Geometry check sheet. Reference: drawing and pictorial views, mm from the part's lowest x, y, z. A direction names the side the tool comes from. Give positions to 0.01 mm unless a question says otherwise; leave off trailing zeros. Loops run counter-clockwise (first coordinate to the right, second up) from the corner with the lowest first, then second, coordinate; pieces in that order, holes last. Notation, with made-up numbers: M 20,-12 L 72,-12 A23 cw 72,24 Z; hole C 64,77.5 d5. An arc over 180 degrees is marked long. Put each result on its own line as item: value. Start each with the question number.
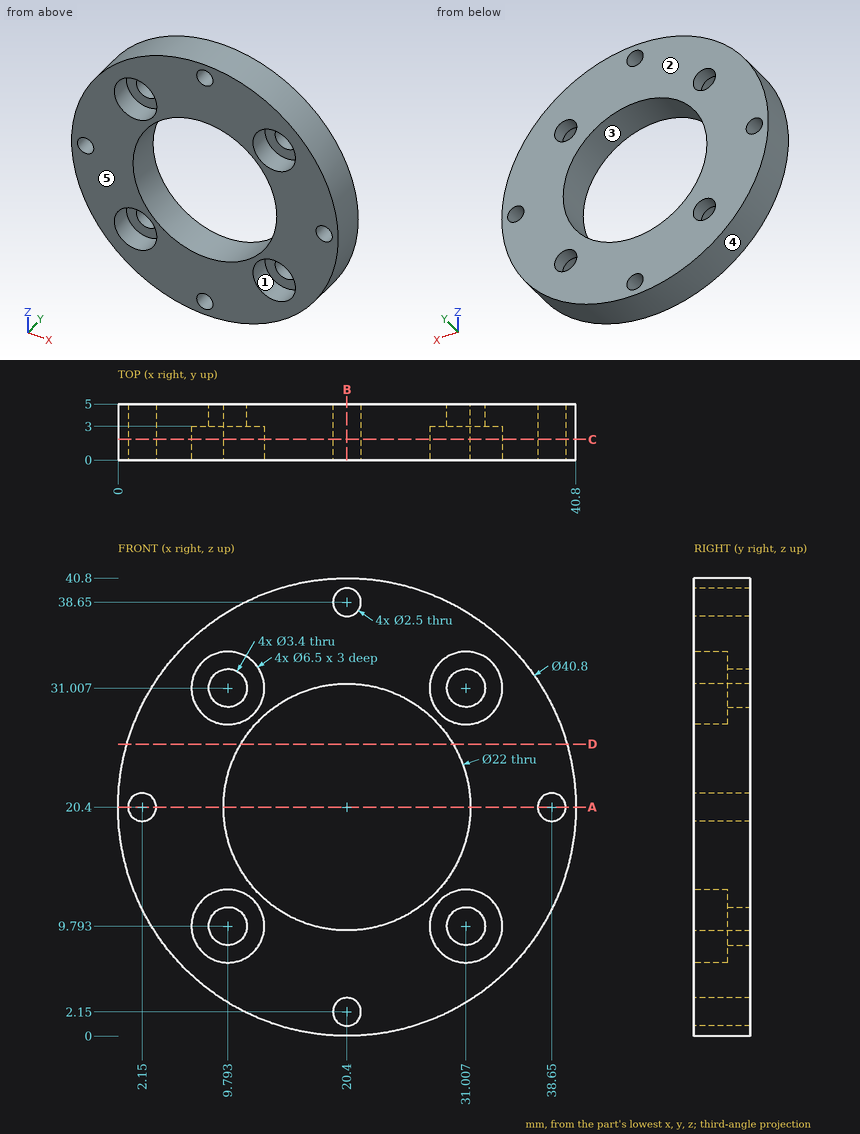
Q1. Section check B-B, the plane x = 20.4. Record the cut outline in (y, z).
Q2. Section check A-A, the plane z = 20.4. Record the cut outline in (x, y).
Q3. Mould release check, pull along Z, two halves, no side actions. Record for the marked faces 3, 4 and 5: pulls with the +Z half, pulls with the -Z half, needs draft (parallel to the pull), parting line crosses it, or undercut.
Q4. Depth check by flat-ended pin: P1, Ø4.5, axis at x = 31.01, z = 9.79, coming from the -Y side; P2, Ø3, axis at y = 4, z = 9.5, coming from the +X side (1 decimal); P3, Ø3, axis at y = 3, z = 14, coming from the -X side. Enter the tip coordinate at first touch or a pass-through.
Q5. Section check D-D, the plane z = 26. Record the cut outline in (x, y).
Q6. Thickness scan on line 1 along X through (y, z) = (3.15, 20.4); line 2 along Z through (x, y) = (7, 2.9) (1 decimal). Record the ranges inside material, lowest first. Write a range as [from, to].
Q7. Access from +Z, -Z, +X, -X, +Y, -Y to the whole of each face (thin tool, end or side, straight path). Record for the marked faces 1 and 2.
Q8. Section check C-C, the plane y = 1.85. Give the number of separate pieces and of enclosed holes in the cut face, then the cut area to 3 significant figures.
Found:
1. outline: M 0,0 L 5,0 L 5,0.9 L 0,0.9 Z; M 0,3.4 L 5,3.4 L 5,9.4 L 0,9.4 Z; M 0,31.4 L 5,31.4 L 5,37.4 L 0,37.4 Z; M 0,39.9 L 5,39.9 L 5,40.8 L 0,40.8 Z
2. outline: M 0,0 L 0.9,0 L 0.9,5 L 0,5 Z; M 3.4,0 L 9.4,0 L 9.4,5 L 3.4,5 Z; M 31.4,0 L 37.4,0 L 37.4,5 L 31.4,5 Z; M 39.9,0 L 40.8,0 L 40.8,5 L 39.9,5 Z
3. face 3: undercut
3. face 4: parting line crosses it
3. face 5: needs draft
4. P1: stops at y = 3
4. P2: stops at x = 38.5
4. P3: stops at x = 0.6
5. outline: M 0.78,0 L 10.93,0 L 10.93,5 L 0.78,5 Z; M 29.87,0 L 40.02,0 L 40.02,5 L 29.87,5 Z
6. line 1: x = [0, 0.9], [3.4, 9.4], [31.4, 37.4], [39.9, 40.8]
6. line 2: z = [5, 8.1], [11.5, 29.3], [32.7, 35.8]
7. face 1: -Y
7. face 2: +Z, -Z, +X, -X, +Y
8. separate pieces: 1
8. enclosed holes: 9
8. area: 775 mm^2
